Verification items for the finished model (mm, model axes). Give positions to 0.01 mm unless a question says otherwise; leave off trailing zeros. Order: outer loops, then holes, each group sorted by start corner. A loop starts at its lowest first (then second) coordinate and runs counter-clockwise, first axis right, second up. Notation, with made-up numbers: (-13.5, 43) - (34.5, 43) arc R12 cw to (34.5, 47) - close; hole circle Ø11 at (62.5, 58.25). An arc over 180 degrees is marked (long way). Answer as a JSON object with one key per item and string values.
```python
from build123d import *

# Parameters (mm, degrees)
SKETCH2_W           = 32
SKETCH2_H           = 62
SKETCH2_R           = 0.305
SKETCH2_R_2         = 2.15265
SKETCH2_R_3         = 1.1303
SKETCH2_W_2         = 23
SKETCH2_H_2         = 18
BOSS_EXTRUDE1_DEPTH = 0.8


with BuildPart() as part:
    # Sketch2 → Boss-Extrude1 (new body)
    with BuildSketch(Plane(origin=(0, 0, 0), x_dir=(1, 0, 0), z_dir=(0, 1, 0))):
        with Locations((16, -31)):
            Rectangle(SKETCH2_W, SKETCH2_H)
        with Locations(Location((9.02, -5.73, 0), (0, 0, 270))):
            Circle(SKETCH2_R, mode=Mode.SUBTRACT)
        with Locations(Location((16, -13, 0), (0, 0, 270))):
            Circle(SKETCH2_R_2, mode=Mode.SUBTRACT)
        with Locations(Location((24.5, -12, 0), (0, 0, 270))):
            Circle(SKETCH2_R_3, mode=Mode.SUBTRACT)
        with Locations(Location((7.5, -12, 0), (0, 0, 270))):
            Circle(SKETCH2_R_3, mode=Mode.SUBTRACT)
        with Locations(Location((8.38, -4.63, 0), (0, 0, 270))):
            Circle(SKETCH2_R, mode=Mode.SUBTRACT)
        with Locations(Location((7.5, -50, 0), (0, 0, 270))):
            Circle(SKETCH2_R_3, mode=Mode.SUBTRACT)
        with Locations(Location((24.5, -50, 0), (0, 0, 270))):
            Circle(SKETCH2_R_3, mode=Mode.SUBTRACT)
        with Locations(Location((16, -49, 0), (0, 0, 270))):
            Circle(SKETCH2_R_2, mode=Mode.SUBTRACT)
        with Locations(Location((9.65, -4.63, 0), (0, 0, 270))):
            Circle(SKETCH2_R, mode=Mode.SUBTRACT)
        with Locations(Location((10.92, -4.63, 0), (0, 0, 270))):
            Circle(SKETCH2_R, mode=Mode.SUBTRACT)
        with Locations(Location((12.19, -4.63, 0), (0, 0, 270))):
            Circle(SKETCH2_R, mode=Mode.SUBTRACT)
        with Locations(Location((13.46, -4.63, 0), (0, 0, 270))):
            Circle(SKETCH2_R, mode=Mode.SUBTRACT)
        with Locations(Location((14.73, -4.63, 0), (0, 0, 270))):
            Circle(SKETCH2_R, mode=Mode.SUBTRACT)
        with Locations(Location((16, -4.63, 0), (0, 0, 270))):
            Circle(SKETCH2_R, mode=Mode.SUBTRACT)
        with Locations(Location((17.27, -4.63, 0), (0, 0, 270))):
            Circle(SKETCH2_R, mode=Mode.SUBTRACT)
        with Locations(Location((18.54, -4.63, 0), (0, 0, 270))):
            Circle(SKETCH2_R, mode=Mode.SUBTRACT)
        with Locations(Location((19.81, -4.63, 0), (0, 0, 270))):
            Circle(SKETCH2_R, mode=Mode.SUBTRACT)
        with Locations(Location((21.08, -4.63, 0), (0, 0, 270))):
            Circle(SKETCH2_R, mode=Mode.SUBTRACT)
        with Locations(Location((22.35, -4.63, 0), (0, 0, 270))):
            Circle(SKETCH2_R, mode=Mode.SUBTRACT)
        with Locations(Location((23.62, -4.63, 0), (0, 0, 270))):
            Circle(SKETCH2_R, mode=Mode.SUBTRACT)
        with Locations(Location((10.29, -5.73, 0), (0, 0, 270))):
            Circle(SKETCH2_R, mode=Mode.SUBTRACT)
        with Locations(Location((11.56, -5.73, 0), (0, 0, 270))):
            Circle(SKETCH2_R, mode=Mode.SUBTRACT)
        with Locations(Location((12.83, -5.73, 0), (0, 0, 270))):
            Circle(SKETCH2_R, mode=Mode.SUBTRACT)
        with Locations(Location((14.1, -5.73, 0), (0, 0, 270))):
            Circle(SKETCH2_R, mode=Mode.SUBTRACT)
        with Locations(Location((15.37, -5.73, 0), (0, 0, 270))):
            Circle(SKETCH2_R, mode=Mode.SUBTRACT)
        with Locations(Location((16.64, -5.73, 0), (0, 0, 270))):
            Circle(SKETCH2_R, mode=Mode.SUBTRACT)
        with Locations(Location((17.91, -5.73, 0), (0, 0, 270))):
            Circle(SKETCH2_R, mode=Mode.SUBTRACT)
        with Locations(Location((19.18, -5.73, 0), (0, 0, 270))):
            Circle(SKETCH2_R, mode=Mode.SUBTRACT)
        with Locations(Location((20.45, -5.73, 0), (0, 0, 270))):
            Circle(SKETCH2_R, mode=Mode.SUBTRACT)
        with Locations(Location((21.72, -5.73, 0), (0, 0, 270))):
            Circle(SKETCH2_R, mode=Mode.SUBTRACT)
        with Locations(Location((22.99, -5.73, 0), (0, 0, 270))):
            Circle(SKETCH2_R, mode=Mode.SUBTRACT)
        with Locations(Location((22.99, -56.27, 0), (0, 0, 270))):
            Circle(SKETCH2_R, mode=Mode.SUBTRACT)
        with Locations(Location((21.72, -56.27, 0), (0, 0, 270))):
            Circle(SKETCH2_R, mode=Mode.SUBTRACT)
        with Locations(Location((20.45, -56.27, 0), (0, 0, 270))):
            Circle(SKETCH2_R, mode=Mode.SUBTRACT)
        with Locations(Location((19.18, -56.27, 0), (0, 0, 270))):
            Circle(SKETCH2_R, mode=Mode.SUBTRACT)
        with Locations(Location((17.91, -56.27, 0), (0, 0, 270))):
            Circle(SKETCH2_R, mode=Mode.SUBTRACT)
        with Locations(Location((16.64, -56.27, 0), (0, 0, 270))):
            Circle(SKETCH2_R, mode=Mode.SUBTRACT)
        with Locations(Location((15.37, -56.27, 0), (0, 0, 270))):
            Circle(SKETCH2_R, mode=Mode.SUBTRACT)
        with Locations(Location((14.1, -56.27, 0), (0, 0, 270))):
            Circle(SKETCH2_R, mode=Mode.SUBTRACT)
        with Locations(Location((12.83, -56.27, 0), (0, 0, 270))):
            Circle(SKETCH2_R, mode=Mode.SUBTRACT)
        with Locations(Location((11.56, -56.27, 0), (0, 0, 270))):
            Circle(SKETCH2_R, mode=Mode.SUBTRACT)
        with Locations(Location((10.29, -56.27, 0), (0, 0, 270))):
            Circle(SKETCH2_R, mode=Mode.SUBTRACT)
        with Locations(Location((23.62, -57.37, 0), (0, 0, 270))):
            Circle(SKETCH2_R, mode=Mode.SUBTRACT)
        with Locations(Location((22.35, -57.37, 0), (0, 0, 270))):
            Circle(SKETCH2_R, mode=Mode.SUBTRACT)
        with Locations(Location((21.08, -57.37, 0), (0, 0, 270))):
            Circle(SKETCH2_R, mode=Mode.SUBTRACT)
        with Locations(Location((19.81, -57.37, 0), (0, 0, 270))):
            Circle(SKETCH2_R, mode=Mode.SUBTRACT)
        with Locations(Location((18.54, -57.37, 0), (0, 0, 270))):
            Circle(SKETCH2_R, mode=Mode.SUBTRACT)
        with Locations(Location((17.27, -57.37, 0), (0, 0, 270))):
            Circle(SKETCH2_R, mode=Mode.SUBTRACT)
        with Locations(Location((16, -57.37, 0), (0, 0, 270))):
            Circle(SKETCH2_R, mode=Mode.SUBTRACT)
        with Locations(Location((14.73, -57.37, 0), (0, 0, 270))):
            Circle(SKETCH2_R, mode=Mode.SUBTRACT)
        with Locations(Location((13.46, -57.37, 0), (0, 0, 270))):
            Circle(SKETCH2_R, mode=Mode.SUBTRACT)
        with Locations(Location((12.19, -57.37, 0), (0, 0, 270))):
            Circle(SKETCH2_R, mode=Mode.SUBTRACT)
        with Locations(Location((10.92, -57.37, 0), (0, 0, 270))):
            Circle(SKETCH2_R, mode=Mode.SUBTRACT)
        with Locations(Location((9.65, -57.37, 0), (0, 0, 270))):
            Circle(SKETCH2_R, mode=Mode.SUBTRACT)
        with Locations(Location((8.38, -57.37, 0), (0, 0, 270))):
            Circle(SKETCH2_R, mode=Mode.SUBTRACT)
        with Locations(Location((9.02, -56.27, 0), (0, 0, 270))):
            Circle(SKETCH2_R, mode=Mode.SUBTRACT)
        with Locations((16, -31)):
            Rectangle(SKETCH2_W_2, SKETCH2_H_2, mode=Mode.SUBTRACT)
    extrude(amount=BOSS_EXTRUDE1_DEPTH)


solid = part.part
```
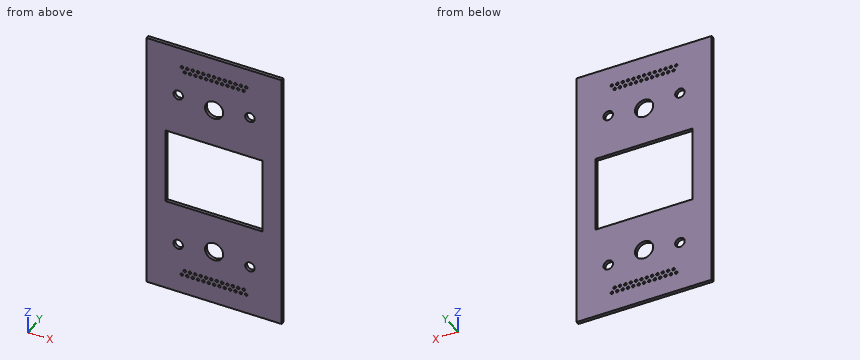
(1) Section check B-B (y = 0.35). Count the separate pieces of the cut face and the enclosed holes in it, then the cut area to 3 significant figures.
Computed values:
{"separate pieces": "1", "enclosed holes": "57", "area": "1,510 mm²"}
(2) Section check A-A (z = 12). Record the cut outline in (x, y), then the cut area to 3 significant figures.
Computed values:
{"outline": "(0, 0) - (6.37, 0) - (6.37, 0.8) - (0, 0.8) - close; (8.63, 0) - (14.09, 0) - (14.09, 0.8) - (8.63, 0.8) - close; (17.91, 0) - (23.37, 0) - (23.37, 0.8) - (17.91, 0.8) - close; (25.63, 0) - (32, 0) - (32, 0.8) - (25.63, 0.8) - close", "area": "18.9 mm²"}
(3) Gauge pin test, flat end, axial feed: pin 1 Ø3 at (x, z) = (7.5, 12) entering from +Y. Record the tip position at first contact, or that the pin passes through.
Computed values:
{"pin 1": "stops at y = 0.8"}
(4) Material ranges on line 1 along Z through (x, y) = (18.54, 0.55) (3 decimals); line 2 along Z through (x, y) = (11.5, 0.2); line 3 along X through (y, z) = (0.55, 23), recorded low to high. Write a range as [from, to].
Computed values:
{"line 1": "z = [0, 4.325], [4.935, 22], [40, 57.065], [57.675, 62]", "line 2": "z = [0, 5.43], [6.03, 22], [40, 55.97], [56.57, 62]", "line 3": "x = [0, 4.5], [27.5, 32]"}
